Geometry: see drawing. Coordinates: mm, zero at the bounding-box minimum. Coordinates: 2 decimals unless noted, no trailing zeros. Order: outer loops, then holes, each group sorted by start corner. A loop starts at its lowest first (then second) coordinate and runs counter-clockwise, first axis right, second up. Notation, with made-up numbers: (31, 62.25) -> (35, 62.25) arc R35 cw to (35, 95.25) -> close; hole circle Ø4 at (70, 23). An arc over 180 degrees is marked (long way). Write each question's results on one line, items separated by ' | '.
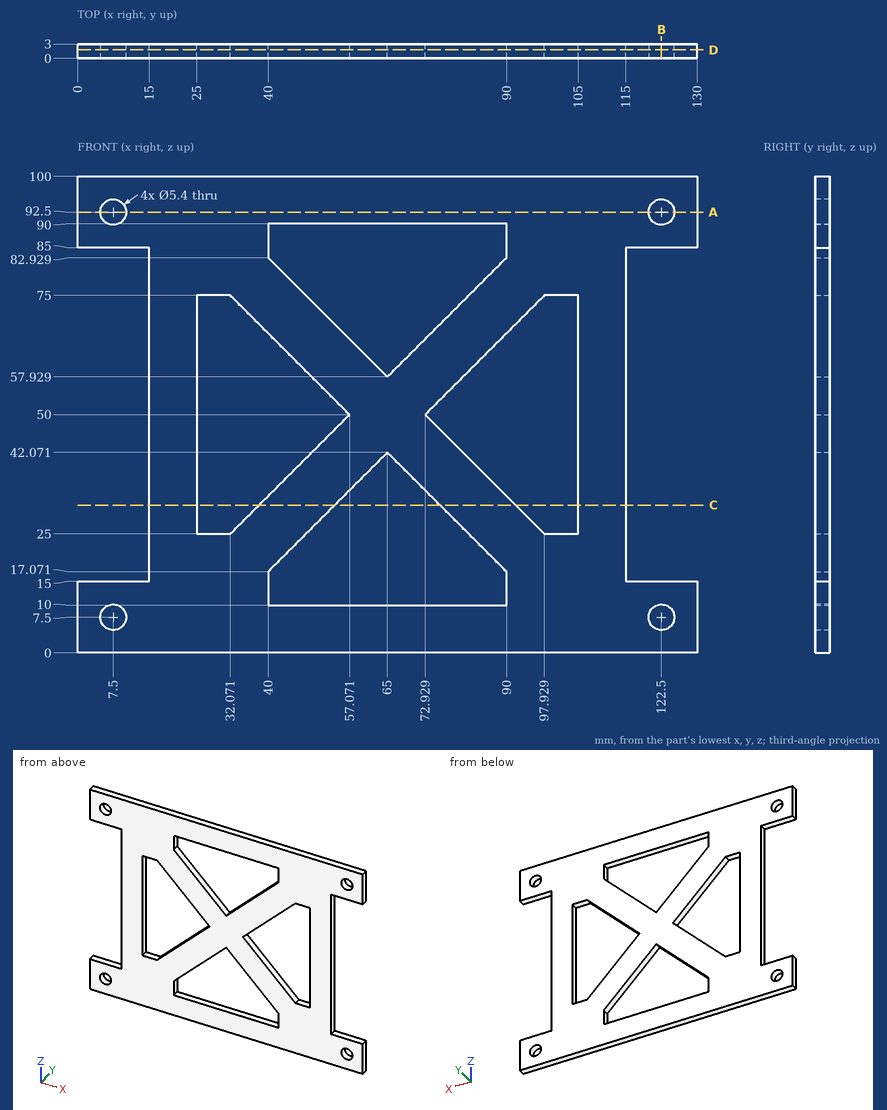
(1) Cut plane C-C, the plane z = 31. Return loops of the section in (x, y), plus the area to 3 significant figures.
Return value:
outline: (15, 0) -> (25, 0) -> (25, 3) -> (15, 3) -> close; (38.07, 0) -> (53.93, 0) -> (53.93, 3) -> (38.07, 3) -> close; (76.07, 0) -> (91.93, 0) -> (91.93, 3) -> (76.07, 3) -> close; (105, 0) -> (115, 0) -> (115, 3) -> (105, 3) -> close | area: 155 mm2
(2) Pin query (flat end, axial travel): P1, Ø0.9, axis at x = 27, y = 1, coming from the -Z side; P2, Ø5, axis at x = 7.5, z = 7.5, coming from the +Y side. Return the tip coordinate at first contact, or that it passes through.
Return value:
P1: z = 0 | P2: through
(3) Cut plane D-D, the plane y = 1.75. Count the separate pieces of the cut face and the enclosed holes in it, plus the area to 3 significant figures.
Return value:
separate pieces: 1 | enclosed holes: 8 | area: 6,890 mm2
(4) Cut plane A-A, the plane z = 92.5. Return loops of the section in (x, y), plus the area to 3 significant figures.
Return value:
outline: (0, 0) -> (4.8, 0) -> (4.8, 3) -> (0, 3) -> close; (10.2, 0) -> (119.8, 0) -> (119.8, 3) -> (10.2, 3) -> close; (125.2, 0) -> (130, 0) -> (130, 3) -> (125.2, 3) -> close | area: 358 mm2
(5) Line query: line 1 along X through (y, z) = (0.9, 92.5); line 2 along Z through (x, y) = (122.5, 1.8); line 3 along X through (y, z) = (0.5, 13.5). Output: solid intervals per line, ascending. Write a range as from..to.
Return value:
line 1: 0..4.8, 10.2..119.8, 125.2..130 | line 2: 0..4.8, 10.2..15, 85..89.8, 95.2..100 | line 3: 0..40, 90..130
(6) Cut plane B-B, the plane x = 122.5. Return loops of the section in (y, z).
Return value:
outline: (0, 0) -> (3, 0) -> (3, 4.8) -> (0, 4.8) -> close; (0, 10.2) -> (3, 10.2) -> (3, 15) -> (0, 15) -> close; (0, 85) -> (3, 85) -> (3, 89.8) -> (0, 89.8) -> close; (0, 95.2) -> (3, 95.2) -> (3, 100) -> (0, 100) -> close
